Source: CAD feature listing. Evaluate the final solid. Frame: model axes, mm. Face numbers are marked on the shaded views. Coordinates: 2 decimals unless noted, no trailing zeros. Order: outer loops, then holes, each group sorted by start corner. A loop starts at its lowest first (then second) coordinate and runs counter-clockwise, first axis right, second up.
Item 1: Section A-A on z = 0. Return the cut outline in (x, y), then the cut area to 3 significant figures.
Item 2: Ray query, line 1 (X direction, y = 11, z = 0); line 2 (Z direction, x = 71, y = 7.5); line 3 (X direction, y = 4.75, z = -7.5). Return the intervals inside material, ascending.
Item 3: Section C-C on y = 4.5. Return the cut outline in (x, z), then the cut area to 3 significant figures.
Item 4: Section B-B on x = 0. Return the cut outline in (y, z).
Item 5: Contact query for flat-ended pins moving along their axis: P1, Ø1, axis at y = 7.5, z = -16.5, coming from the +X side; P2, Ø6, axis at x = 55.5, z = 64, coming from the +Y side; P3, Ø6, axis at y = 10, z = -28.5, coming from the +X side. Output: stop coordinate, or through.
Item 6: Mould query, pull axis Z, two halves, no side actions, for the marked faces 1, 2 and 3. Classes: released by +Z, released by -Z, zero draft, split by the parting line, or undercut.
from build123d import *

# Parameters (mm, degrees)
SKETCH_1_R      = 90
SKETCH_1_R_2    = 80
EXTRUDE_1_DEPTH = 7
SKETCH_1_3_R    = 92.5
SKETCH_1_3_R_2  = 90
SKETCH_1_3_R_3  = 80
SKETCH_1_3_R_4  = 77.5
EXTRUDE_2_DEPTH = 14


with BuildPart() as part:
    # Sketch 1 → Extrude 1 (new body)
    with BuildSketch(Plane(origin=(0, 0, 0), x_dir=(1, 0, 0), z_dir=(0, 1, 0))):
        with Locations(Location((0, 0, 0), (0, 0, 270))):
            Circle(SKETCH_1_R)
        with Locations(Location((0, 0, 0), (0, 0, 270))):
            Circle(SKETCH_1_R_2, mode=Mode.SUBTRACT)
    extrude(amount=EXTRUDE_1_DEPTH)

    # Sketch 1_3 → Extrude 2 (add)
    # profile 1 of 2: a face of its own
    with BuildSketch(Plane(origin=(0, 0, 0), x_dir=(1, 0, 0), z_dir=(0, 1, 0))):
        with Locations(Location((0, 0, 0), (0, 0, 270))):
            Circle(SKETCH_1_3_R)
        with Locations(Location((0, 0, 0), (0, 0, 270))):
            Circle(SKETCH_1_3_R_2, mode=Mode.SUBTRACT)
    # profile 2 of 2: a face of its own
    with BuildSketch(Plane(origin=(0, 0, 0), x_dir=(1, 0, 0), z_dir=(0, 1, 0))):
        with Locations(Location((0, 0, 0), (0, 0, 270))):
            Circle(SKETCH_1_3_R_3)
        with Locations(Location((0, 0, 0), (0, 0, 270))):
            Circle(SKETCH_1_3_R_4, mode=Mode.SUBTRACT)
    extrude(amount=EXTRUDE_2_DEPTH)

    # Sweep 1: sweep along a path in Sketch 3
    with BuildLine(Plane(origin=(0, 7, 0), x_dir=(1, 0, 0), z_dir=(0, 1, 0))) as sweep_1_path:
        CenterArc((0, 0), 85, 0, 360)
    # Sketch 2 → Sweep 1 (sweep, cut)
    with BuildSketch(Plane.XY):
        with BuildLine():
            Line((-90, 7), (-80, 7))
            ThreePointArc((-80, 7), (-85, 2), (-90, 7))
        make_face()
    sweep(path=sweep_1_path.line, mode=Mode.SUBTRACT)


solid = part.part
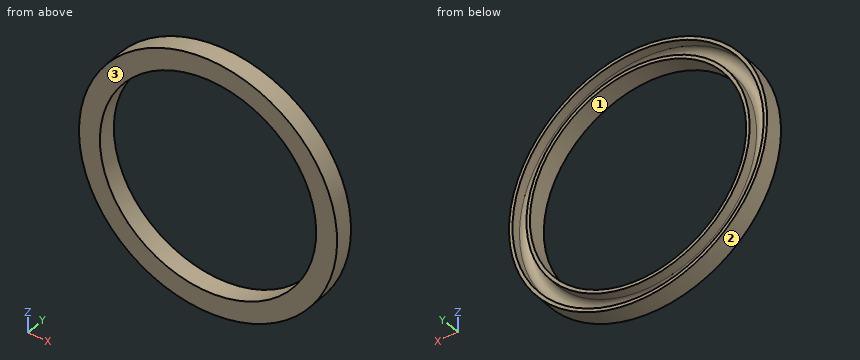
Answer list:
1. outline: (-92.5, 0) - (-77.5, 0) - (-77.5, 14) - (-80, 14) - (-80, 7) arc R5 cw to (-90, 7) - (-90, 14) - (-92.5, 14) - close; (77.5, 0) - (92.5, 0) - (92.5, 14) - (90, 14) - (90, 7) arc R5 cw to (80, 7) - (80, 14) - (77.5, 14) - close
1. area: 201 mm2
2. line 1: x = -92.5 to -90, -80 to -77.5, 77.5 to 80, 90 to 92.5
2. line 2: z = -59.29 to -55.31, -36.86 to -31.07, 31.07 to 36.86, 55.31 to 59.29
2. line 3: x = -92.2 to -89.15, -80.18 to -77.14, 77.14 to 80.18, 89.15 to 92.2
3. outline: circle Ø185 at (0, 0); circle Ø161.34 at (0, 0); hole circle Ø178.66 at (0, 0); hole circle Ø155 at (0, 0)
3. area: 3,390 mm2
4. outline: (0, -92.5) - (14, -92.5) - (14, -90) - (7, -90) arc R5 cw to (7, -80) - (14, -80) - (14, -77.5) - (0, -77.5) - close; (0, 77.5) - (14, 77.5) - (14, 80) - (7, 80) arc R5 cw to (7, 90) - (14, 90) - (14, 92.5) - (0, 92.5) - close
5. P1: stops at x = 91.11
5. P2: stops at y = 3.23
5. P3: stops at x = 88.92
6. face 1: undercut
6. face 2: split by the parting line
6. face 3: zero draft
